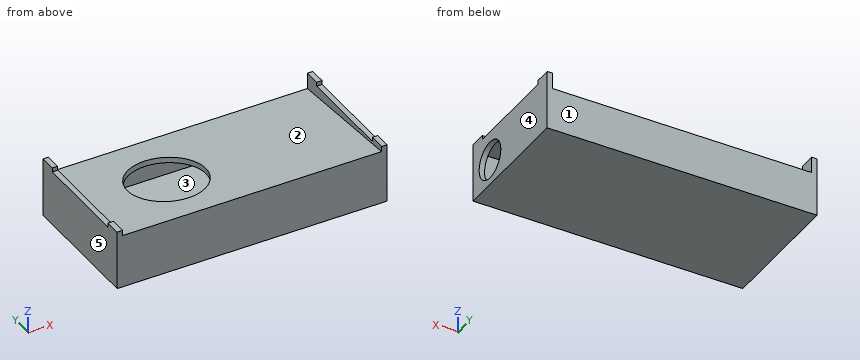
from build123d import *

# Parameters (mm, degrees)
F0_W      = 635
F0_H      = 304.8
F1_DEPTH  = 127
F3_DEPTH  = 635.001
F4_T      = -12.7
F5_R      = 89.535
F6_DEPTH  = 12.7
F8_D      = 88.9
F8_DEPTH  = 25.4
F8_TIP    = 26.7082545158
F10_DEPTH = 12.7
F12_DEPTH = 12.7


with BuildPart() as f1:
    # F0 (on Top) → F1 (new body)
    with BuildSketch(Plane.XY):
        Rectangle(F0_W, F0_H)
    extrude(amount=F1_DEPTH)

    # F2 (on face) → F3 (cut, through all)
    with BuildSketch(Plane.YZ.offset(317.5)):
        Polygon((-152.4, 127), (152.4, 101.6), (152.4, 127), align=None)
    extrude(amount=-F3_DEPTH, mode=Mode.SUBTRACT)

    # F4 (hollow: no face is removed)
    offset(amount=F4_T, mode=Mode.SUBTRACT)

    # F5 (on face) → F6 (cut, through all)
    with BuildSketch(Plane(origin=(0, 9.4593103448, 113.5117241379), x_dir=(1, 0, 0), z_dir=(0, 0.0830454799, 0.9965457582))):
        with Locations((-117.475, -15.3138471966)):
            Circle(F5_R)
    extrude(amount=-F6_DEPTH, mode=Mode.SUBTRACT)

    # F8
    with Locations(Plane.YZ.offset(317.5)):
        with Locations((-82.6105548445, 60.5921064519)):
            Hole(F8_D / 2, depth=F8_DEPTH)
            with Locations((0, 0, -(F8_DEPTH + F8_TIP / 2))):  # 118° drill point
                Cone(0, F8_D / 2, F8_TIP, mode=Mode.SUBTRACT)

    # F9 (on face) → F10 (join)
    with BuildSketch(Plane.YZ.offset(317.5)):
        Polygon((-152.4, 139.7), (-152.4, 127), (152.4, 101.6), (152.4, 139.7), (114.3, 139.7), (114.3, 130.104392767), (-114.3, 130.104392767), (-114.3, 139.7), align=None)
    extrude(amount=-F10_DEPTH)

    # F11 (on face) → F12 (join)
    with BuildSketch(Plane(origin=(-317.5, 0, 0), x_dir=(0, -1, 0), z_dir=(-1, 0, 0))):
        Polygon((-152.4, 139.7), (-152.4, 101.6), (152.4, 127), (152.4, 139.7), (114.3, 139.7), (114.3, 130.104392767), (-114.3, 130.104392767), (-114.3, 139.7), align=None)
    extrude(amount=-F12_DEPTH)


solid = f1.part
The listing builds one solid part. Answer for the finished solid, in the listing's coordinates (mm). Face numbers are marked on the shaded views. A direction names the side the tool comes from. Give positions to 0.01 mm unless a question says otherwise; leave off trailing zeros. Loops run counter-clockwise (first coordinate to the right, second up) from the corner with the lowest first, then second, coordinate; pieces in that order, holes last.
Item 1: Determine the mould class of the marked faces 3, 4 and 5 for opening direction X: +X half, -X half, draft (parallel to the pull), parting line (faces both ways), or undercut.
Derived:
face 3: undercut
face 4: +X half
face 5: -X half
Item 2: A cutting plane is placed at D-D (x = -189). Give the vertices of the cut face in (y, z), then the cut area to 3 significant figures.
Derived:
outline: (-152.4, 0) - (152.4, 0) - (152.4, 101.6) - (47.87, 110.31) - (46.82, 97.65) - (139.7, 89.91) - (139.7, 12.7) - (-139.7, 12.7) - (-139.7, 113.2) - (-60.53, 106.6) - (-59.47, 119.26) - (-152.4, 127) - close
area: 8,640 mm2
Item 3: A cutting plane is placed at A-A (x = 185.5). Give the vertices of the cut face in (y, z), then the cut area to 3 significant figures.
Derived:
outline: (-152.4, 0) - (152.4, 0) - (152.4, 101.6) - (-152.4, 127) - close; hole (-139.7, 12.7) - (139.7, 12.7) - (139.7, 89.91) - (-139.7, 113.2) - close
area: 10,000 mm2
Item 4: Each of these flat-tipped pins is pushed along its axis until it touches: pin 1 Ø3 at (x, y) = (201.5, 10.5) entering from +Z; pin 2 Ø12 at (y, z) = (-98.5, 37.5) entering from +X; pin 3 Ø5 at (x, y) = (127, 37.5) entering from +Z. Where does it stop, or does it pass through?
Derived:
pin 1: stops at z = 113.55
pin 2: stops at x = -304.8
pin 3: stops at z = 111.38
Item 5: Find the intervals of material crossed by line 1 along Y through (x, z) = (35, 54.5); line 2 along X through (y, z) = (-96.5, 106); line 3 along X through (y, z) = (-63.5, 56), in increasing order.
Derived:
line 1: y = -152.4 to -139.7, 139.7 to 152.4
line 2: x = -317.5 to -304.8, 304.8 to 317.5
line 3: x = -317.5 to -304.8
Item 6: A cutting plane is placed at C-C (z = 45.5). Give the vertices of the cut face in (x, y).
Derived:
outline: (-317.5, -152.4) - (317.5, -152.4) - (317.5, -124.42) - (304.8, -124.42) - (304.8, -139.7) - (-304.8, -139.7) - (-304.8, 139.7) - (304.8, 139.7) - (304.8, -40.8) - (317.5, -40.8) - (317.5, 152.4) - (-317.5, 152.4) - close
Item 7: A cutting plane is placed at B-B (y = 127.5). Give the vertices of the cut face in (x, z) (3 decimals), then the cut area to 3 significant figures.
Derived:
outline: (-317.5, 0) - (317.5, 0) - (317.5, 139.7) - (304.8, 139.7) - (304.8, 103.675) - (-304.8, 103.675) - (-304.8, 139.7) - (-317.5, 139.7) - close; hole (-304.8, 12.7) - (304.8, 12.7) - (304.8, 90.931) - (-304.8, 90.931) - close
area: 19,100 mm2
Item 8: A tool of negligible diameter and unlimited length cuts with its end or side. For the marked faces 1 and 2, from which of +Z, -Z, +X, -X, +Y, -Y can it reach the whole face along a straight path? Write none if from no direction.
Derived:
face 1: +Z, -Z, +X, -X, +Y
face 2: +Z, +Y
